from build123d import *

# Parameters (mm, degrees)
F1_DEPTH = 6
F3_DEPTH = 25
F4_R     = 5


with BuildPart() as f1:
    # F0 (on Top) → F1 (new body)
    with BuildSketch(Plane.XY):
        with BuildLine():
            Line((-1, 0), (0, 0))
            Line((0, 0), (5, 0))
            Line((5, 0), (5, 17))
            Line((5, 17), (-26, 17))
            Line((-26, 17), (-26, 9))
            Line((-26, 9), (0, 9))
            Line((0, 9), (0, 3))
            Line((0, 3), (-1, 3))
            ThreePointArc((-1, 3), (-2.5, 1.5), (-1, 0))
        make_face()
    extrude(amount=F1_DEPTH)

    # F2 (on face) → F3 (cut)
    with BuildSketch(Plane(origin=(0, 17, 0), x_dir=(-1, 0, 0), z_dir=(0, 1, 0))):
        with BuildLine():
            ThreePointArc((22.75, 1.25), (23.9874368671, 1.7625631329), (24.5, 3))
            ThreePointArc((24.5, 3), (23.9874368671, 4.2374368671), (22.75, 4.75))
            Line((22.75, 4.75), (22.75, 1.25))
        make_face()
        with BuildLine():
            Line((22.75, 1.25), (22.75, 4.75))
            ThreePointArc((22.75, 4.75), (22.2259514134, 4.6696925103), (21.75, 4.4361406616))
            ThreePointArc((21.75, 4.4361406616), (22.3012092057, 3.8100925873), (22.5, 3))
            ThreePointArc((22.5, 3), (22.3012092057, 2.1899074127), (21.75, 1.5638593384))
            ThreePointArc((21.75, 1.5638593384), (22.2259514134, 1.3303074897), (22.75, 1.25))
        make_face()
        with BuildLine():
            ThreePointArc((21.75, 4.4361406616), (22.2259514134, 4.6696925103), (22.75, 4.75))
            Line((22.75, 4.75), (20.75, 4.75))
            ThreePointArc((20.75, 4.75), (21.2740485866, 4.6696925103), (21.75, 4.4361406616))
        make_face()
        with BuildLine():
            Line((20.75, 1.25), (22.75, 1.25))
            ThreePointArc((22.75, 1.25), (22.2259514134, 1.3303074897), (21.75, 1.5638593384))
            ThreePointArc((21.75, 1.5638593384), (21.2740485866, 1.3303074897), (20.75, 1.25))
        make_face()
        with BuildLine():
            ThreePointArc((21.75, 1.5638593384), (21, 3), (21.75, 4.4361406616))
            ThreePointArc((21.75, 4.4361406616), (21.2740485866, 4.6696925103), (20.75, 4.75))
            ThreePointArc((20.75, 4.75), (19, 3), (20.75, 1.25))
            ThreePointArc((20.75, 1.25), (21.2740485866, 1.3303074897), (21.75, 1.5638593384))
        make_face()
        with BuildLine():
            ThreePointArc((22.5, 3), (22.3012092057, 3.8100925873), (21.75, 4.4361406616))
            ThreePointArc((21.75, 4.4361406616), (21, 3), (21.75, 1.5638593384))
            ThreePointArc((21.75, 1.5638593384), (22.3012092057, 2.1899074127), (22.5, 3))
        make_face()
    extrude(amount=-F3_DEPTH, mode=Mode.SUBTRACT)

    # F4
    f4_edges = [f1.edges().sort_by_distance(p)[0] for p in [
        (5, 17, 3),
        (5, 0, 3),
    ]]
    fillet(f4_edges, radius=F4_R)


solid = f1.part
Read the model definition and answer for the solid it produces. Units are mm, in the model's axes. A direction names the side the tool comes from. Round coordinates to 2 decimals unless told otherwise and drop trailing zeros. Write each loop counter-clockwise with the first axis right and the second up, starting at its lowest first coordinate (ties: lowest second). Pieces come first, ordered by that corner, then holes.
Q1. The mould has two halves that part along Y. Classify faces 1 (the face through (-0.5, 0, 3)), 2 (the face through (-0.5, 3, 3)), 3 (the face through (0, 6, 3)), 4 (the face through (-26, 13, 3)): released by +Y, released by -Y, zero draft, split by the parting line, or undercut.
Values:
face 1: released by -Y
face 2: undercut
face 3: undercut
face 4: zero draft
Q2. Find section B-B on z = 0.5. Determine the outline of the cut face in (x, y).
Values:
outline: (-26, 9) - (0, 9) - (0, 3) - (-1, 3) arc R1.5 ccw to (-1, 0) - (0, 0) arc R5 ccw to (5, 5) - (5, 12) arc R5 ccw to (0, 17) - (-26, 17) - close
Q3. Find section C-C on y = 15. Determine the outline of the cut face in (x, z), and give its area (3 significant figures).
Values:
outline: (-26, 0) - (4, 0) - (4, 6) - (-26, 6) - close; hole (-22.75, 1.25) - (-20.75, 1.25) arc R1.75 ccw to (-20.75, 4.75) - (-22.75, 4.75) arc R1.75 ccw to start
area: 163 mm2
Q4. Flat-ended cylindrical pins translate along their axes: P1, Ø3, axis at y = 7, z = 3, coming from the -X side; P2, Ø2, axis at x = -22, y = 14, coming from the -Z side; P3, Ø3, axis at x = -19, z = 1.5, coming from the -Y side. Find the tip coordinate at first contact, or state that the pin passes through.
Values:
P1: stops at x = 0
P2: stops at z = 0
P3: stops at y = 9
Q5. Find section A-A on x = -21.5. Determine the outline of the cut face in (y, z), and give its area (3 significant figures).
Values:
outline: (9, 0) - (17, 0) - (17, 1.25) - (9, 1.25) - close; (9, 4.75) - (17, 4.75) - (17, 6) - (9, 6) - close
area: 20.0 mm2
Q6. Straight lines are drawn through the part: line 1 (Y direction, x = -14.5, z = 4.3); line 2 (X direction, y = 14.25, z = 3.65); line 3 (X direction, y = 9.25, z = 4.05). For each, find the intervals that lie inside material, in ascending order.
Values:
line 1: y = 9 to 17
line 2: x = -26 to -24.37, -19.13 to 4.47
line 3: x = -26 to -24.15, -19.35 to 5
Q7. Find section D-D on z = 4.3. Determine the outline of the cut face in (x, y).
Values:
outline: (-26, 9) - (-23.92, 9) - (-23.92, 17) - (-26, 17) - close; (-19.58, 9) - (0, 9) - (0, 3) - (-1, 3) arc R1.5 ccw to (-1, 0) - (0, 0) arc R5 ccw to (5, 5) - (5, 12) arc R5 ccw to (0, 17) - (-19.58, 17) - close
Q8. A tool of negligible diameter and unlimited length cuts with its end or side. For faces 5 (the face through (-22, 13, 1.25)), 6 (the face through (3, 1, 3)), from which of +Z, -Z, +X, -X, +Y, -Y can it reach the whole face along a straight path? Write none if from no direction.
Values:
face 5: +Y, -Y
face 6: +Z, -Z, +X, -Y
